The model under review builds one solid part; all positions refer to its coordinate system, in mm. A direction names the side the tool comes from. Give positions to 0.01 mm unless a question says otherwise; leave off trailing zeros. Order: outer loops, then holes, each group sorted by start corner. A loop starts at its lowest first (then second) coordinate and runs counter-clockwise, first axis right, second up. Notation, with made-up numbers: (-29, 35) - (-3, 35) arc R21 cw to (-3, 51) - close; hole circle Ø8 at (44.25, 10.5). An arc over 180 degrees is marked (long way). Use CSV: the item, a comma, the result in double quotes.
```python
from build123d import *

# Parameters (mm, degrees)
F0_R            = 100
F1_DEPTH        = 25
F3_DEPTH        = 25
F3_COPIES_COUNT = 20
F4_SIZE         = 2
F5_R            = 5
F6_R            = 90
F7_DEPTH        = 5
F8_R            = 30
F8_R_2          = 15
F9_DEPTH        = 30


# Not quite as in the source:
# - a pattern or mirror of a feature is missing from the dataset's text; its kind, count and spacing are read off the source's solid


with BuildPart() as f1:
    # F0 (on Front) → F1 (new body)
    with BuildSketch(Plane.XZ):
        Circle(F0_R)
    extrude(amount=F1_DEPTH)

    # F2 (on face) → F3 (join)
    with BuildSketch(Plane.XZ.offset(25)):
        Polygon((-4.5, 120), (-9.9931095726, 99.4994359837), (9.9931095726, 99.4994359837), (4.5, 120), align=None)
    f3 = extrude(amount=-F3_DEPTH)

    # F3_copies: F3 ×20 about axis
    f3_copies_axis = Axis((0, 0, 0), (0, 1, 0))
    for i in range(1, F3_COPIES_COUNT):
        add(f3.rotate(f3_copies_axis, i * 360 / F3_COPIES_COUNT))

    # F4
    f4_edges = [f1.edges().sort_by_distance(p)[0] for p in [
        (4.5, -12.5, 120),
        (-4.5, -12.5, 120),
        (-32.802285, -12.5, 115.517358),
        (115.517358, -12.5, 32.802285),
        (120, -12.5, 4.5),
        (120, -12.5, -4.5),
        (115.517358, -12.5, -32.802285),
        (112.736205, -12.5, -41.361794),
        (99.727073, -12.5, -66.893654),
        (94.437006, -12.5, -74.174807),
        (74.174807, -12.5, -94.437006),
        (66.893654, -12.5, -99.727073),
        (41.361794, -12.5, -112.736205),
        (32.802285, -12.5, -115.517358),
        (4.5, -12.5, -120),
        (-4.5, -12.5, -120),
        (-32.802285, -12.5, -115.517358),
        (-41.361794, -12.5, -112.736205),
        (-66.893654, -12.5, -99.727073),
        (-74.174807, -12.5, -94.437006),
        (-94.437006, -12.5, -74.174807),
        (-99.727073, -12.5, -66.893654),
        (-112.736205, -12.5, -41.361794),
        (-115.517358, -12.5, -32.802285),
        (-120, -12.5, -4.5),
        (-120, -12.5, 4.5),
        (-115.517358, -12.5, 32.802285),
        (-112.736205, -12.5, 41.361794),
        (-99.727073, -12.5, 66.893654),
        (-94.437006, -12.5, 74.174807),
        (-74.174807, -12.5, 94.437006),
        (-66.893654, -12.5, 99.727073),
        (32.802285, -12.5, 115.517358),
        (41.361794, -12.5, 112.736205),
        (66.893654, -12.5, 99.727073),
        (74.174807, -12.5, 94.437006),
        (94.437006, -12.5, 74.174807),
        (99.727073, -12.5, 66.893654),
        (112.736205, -12.5, 41.361794),
        (-41.361794, -12.5, 112.736205),
    ]]
    chamfer(f4_edges, length=F4_SIZE)

    # F5
    f5_edges = [f1.edges().sort_by_distance(p)[0] for p in [
        (9.99311, -12.5, 99.499436),
        (-9.99311, -12.5, 99.499436),
        (97.717628, -12.5, 21.243005),
        (99.499436, -12.5, 9.99311),
        (91.541546, -12.5, 40.251029),
        (86.370537, -12.5, 50.399706),
        (99.499436, -12.5, -9.99311),
        (97.717628, -12.5, -21.243005),
        (74.622932, -12.5, 66.568897),
        (66.568897, -12.5, 74.622932),
        (91.541546, -12.5, -40.251029),
        (86.370537, -12.5, -50.399706),
        (50.399706, -12.5, 86.370537),
        (40.251029, -12.5, 91.541546),
        (74.622932, -12.5, -66.568897),
        (66.568897, -12.5, -74.622932),
        (21.243005, -12.5, 97.717628),
        (50.399706, -12.5, -86.370537),
        (40.251029, -12.5, -91.541546),
        (-21.243005, -12.5, 97.717628),
        (21.243005, -12.5, -97.717628),
        (9.99311, -12.5, -99.499436),
        (-40.251029, -12.5, 91.541546),
        (-50.399706, -12.5, 86.370537),
        (-9.99311, -12.5, -99.499436),
        (-21.243005, -12.5, -97.717628),
        (-66.568897, -12.5, 74.622932),
        (-74.622932, -12.5, 66.568897),
        (-40.251029, -12.5, -91.541546),
        (-50.399706, -12.5, -86.370537),
        (-86.370537, -12.5, 50.399706),
        (-91.541546, -12.5, 40.251029),
        (-66.568897, -12.5, -74.622932),
        (-74.622932, -12.5, -66.568897),
        (-97.717628, -12.5, 21.243005),
        (-99.499436, -12.5, 9.99311),
        (-86.370537, -12.5, -50.399706),
        (-91.541546, -12.5, -40.251029),
        (-99.499436, -12.5, -9.99311),
        (-97.717628, -12.5, -21.243005),
    ]]
    fillet(f5_edges, radius=F5_R)

    # F6 (on face) → F7 (cut)
    with BuildSketch(Plane.XZ.offset(25)):
        Circle(F6_R)
    extrude(amount=-F7_DEPTH, mode=Mode.SUBTRACT)

    # F8 (on face) → F9 (join)
    with BuildSketch(Plane.XZ.offset(20)):
        Circle(F8_R)
        Circle(F8_R_2, mode=Mode.SUBTRACT)
    extrude(amount=F9_DEPTH)


solid = f1.part
```
Item 1: Take a section at A-A, the plane y = -32. Give the boundary of the cut face in (x, z), and give its area (3 significant figures).
Results list:
outline,"circle Ø60 at (0, 0); hole circle Ø30 at (0, 0)"
area,"2,120 mm2"
Item 2: Wall thickness on L1, parallel to Z at x = 0, y = -37.5; L2, parallel to Z at x = 0, y = -22; L3, parallel to Z at x = 101, y = -15: over which ranges is each line inside the solid? List them lowest first.
Results list:
L1,"z = -30 to -15, 15 to 30"
L2,"z = -120 to -90, -30 to -15, 15 to 30, 90 to 120"
L3,"z = -40.75 to -23.37, -10 to 10, 23.37 to 40.75"
Item 3: Take a section at B-B, the plane x = 59.5. Give the boundary of the cut face in (y, z), and give its area (3 significant figures).
Results list:
outline,"(-25, -93.74) - (0, -93.74) - (0, 93.74) - (-25, 93.74) - (-25, 67.53) - (-20, 67.53) - (-20, -67.53) - (-25, -67.53) - close"
area,"4,010 mm2"
Item 4: Tool access review of faces 4 (the face through (-29.97, -34.79, 1.32)), 5 (the face through (59.101, -12.675, -93.417)), 6 (the face through (-107.29, -12.68, 27.46)), 7 (the face through (93.557, -12.675, -59.274)), 8 (the face through (40.837, -12.675, 102.723)): name each direction out of +Z, -Z, +X, -X, +Y, -Y from which nothing blocks a thin tool from reaching the whole face with its end or side.
Results list:
face 4,"-Y"
face 5,"-Z, +Y, -Y"
face 6,"-X, +Y, -Y"
face 7,"+X, +Y, -Y"
face 8,"+Y, -Y"
Item 5: Mouldability with a two-part tool opening along Z and no side actions: class faces 1 (the face through (7.1, -12.7, 110.3)), 2 (the face through (74.86, -12.325, 67.584)), 3 (the face through (50.393, -12.325, -87.416)) as pulls with the +Z half, pulls with the -Z half, needs draft (parallel to the pull), parting line crosses it, or undercut.
Results list:
face 1,"pulls with the +Z half"
face 2,"undercut"
face 3,"pulls with the -Z half"
Item 6: Take a section at C-C, the plane z = -56. Give the boundary of the cut face in (x, y).
Results list:
outline,"(-90.91, -25) - (-70.46, -25) - (-70.46, -20) - (70.46, -20) - (70.46, -25) - (90.91, -25) - (90.91, 0) - (-90.91, 0) - close"
Item 7: Clearance check with flat-ended pins moving along their axes: pin 1 (10 mm diameter, centred on x = -16.5, y = -29, fed in from +Z); pin 2 (3 mm diameter, centred on x = 69, z = 59.5, fed in from -Y); pin 3 (1 mm diameter, centred on y = -6.5, z = 95.5, fed in from +X). State where each tip first meets the part, or that it passes through.
Results list:
pin 1,"stops at z = 99.08"
pin 2,"stops at y = -25"
pin 3,"stops at x = 72.74"
